Can you work these out from the model? Positions are in its coordinate system, mm. Give positions to 0.01 mm unless a question says otherwise; leave off trailing zeros. Order: outer loops, then holes, each group sorted by start corner. A loop starts at its lowest first (then second) coordinate and runs counter-clockwise, first axis right, second up. Notation, with made-up numbers: M 10,-34.5 L 62,-34.5 A21 cw 62,-25.5 Z; hole C 10.25,80.5 d11. An arc over 180 degrees is marked long. Use one line per item in the form item = value. Start each with the question number.
1. I need wall thicknesses on L1, parallel to Y at x = 0, z = 26.5; L2, parallel to Y at x = 0, z = 12; L3, parallel to Z at x = -11.5, y = -9.5. Which ranges of each line are inside material? Lowest first, please.
2. Will these pins go through, and if not, where does the flat tip stop? P1, Ø8, axis at x = -12, z = 13, coming from the -Y side; P2, Ø6, axis at x = 9.5, y = 14, coming from the -Z side; P3, Ø12, axis at y = -17, z = 24.5, coming from the -X side; P4, Ø2.5, axis at x = 0, y = 19.13, coming from the +Z side.
3. I want a section at D-D, the plane z = 3.75. List the corners of the cut face in (x, y) for me.
4. I want a section at B-B, the plane x = -19. List the corners of the cut face in (y, z) for me, and give its area (3 significant figures).
5. I want a section at A-A, the plane y = 0. List the corners of the cut face in (x, z) for me, and give its area (3 significant figures).
6. We'd pull the mould along X, two halves only. Please class faces 1 (the face through (-2.38, -10.74, 12.32)), 2 (the face through (-1.73, -7.81, 14.3)), 3 (the face through (10, 5, 25)): +X half, -X half, draft (parallel to the pull), parting line (faces both ways), or undercut.
7. I want a section at C-C, the plane x = -1.5. List the corners of the cut face in (y, z) for me.
```python
from build123d import *

# Parameters (mm, degrees)
F0_R     = 11
F0_R_2   = 8
F1_DEPTH = 25
F2_R     = 22.5
F2_R_2   = 11
F2_R_3   = 8
F3_DEPTH = 4
F5_D     = 4.4


with BuildPart() as f1:
    # F0 (on Top) → F1 (new body)
    with BuildSketch(Plane.XY):
        Circle(F0_R)
        Circle(F0_R_2, mode=Mode.SUBTRACT)
    extrude(amount=F1_DEPTH)

    # F2 (on face) → F3 (join)
    with BuildSketch(Plane.XY.offset(25)):
        Circle(F2_R)
        Circle(F2_R_2, mode=Mode.SUBTRACT)
        Circle(F2_R_2)
        Circle(F2_R_3, mode=Mode.SUBTRACT)
    extrude(amount=F3_DEPTH)

    # F5 (through all)
    with Locations(Plane.XY.offset(29)):
        with Locations((-19, 0), (0, 19.126665961), (19, 0), (0, -18.3666665865)):
            Hole(F5_D / 2)


solid = f1.part
```
Check result:
q1.L1 = -22.5 to -20.57, -16.17 to -8, 8 to 16.93, 21.33 to 22.5
q1.L2 = -11 to -8, 8 to 11
q1.L3 = 25 to 29
q2.P1 = -7.55
q2.P2 = 25
q2.P3 = -19.62
q2.P4 = through
q3.outline = C 0,0 d22; hole C 0,0 d16
q4.outline = M -12.05,25 L -2.2,25 L -2.2,29 L -12.05,29 Z; M 2.2,25 L 12.05,25 L 12.05,29 L 2.2,29 Z
q4.area = 78.8 mm2
q5.outline = M -22.5,25 L -21.2,25 L -21.2,29 L -22.5,29 Z; M -16.8,25 L -11,25 L -11,0 L -8,0 L -8,29 L -16.8,29 Z; M 8,0 L 11,0 L 11,25 L 16.8,25 L 16.8,29 L 8,29 Z; M 21.2,25 L 22.5,25 L 22.5,29 L 21.2,29 Z
q5.area = 231 mm2
q6.face_1 = parting line
q6.face_2 = undercut
q6.face_3 = draft
q7.outline = M -22.45,25 L -19.98,25 L -19.98,29 L -22.45,29 Z; M -16.76,25 L -10.9,25 L -10.9,0 L -7.86,0 L -7.86,29 L -16.76,29 Z; M 7.86,0 L 10.9,0 L 10.9,25 L 17.52,25 L 17.52,29 L 7.86,29 Z; M 20.74,25 L 22.45,25 L 22.45,29 L 20.74,29 Z
